Design review of the part shown in the three views and the two pictorial views. Dimensions are in mm from the part's minimum x, y and z. Coordinates: 2 decimals unless noted, no trailing zeros. Write each loop counter-clockwise with the first axis right and the second up, starting at its lowest first coordinate (ties: lowest second). Pieces come first, ordered by that corner, then holes.
Q1. The part is to be moulded in two halves that separate along Y. For the marked faces 1, 2, 3 and 4, say which applies: released by +Y, released by -Y, zero draft, split by the parting line, or undercut.
Q2. For L1, parallel to Y at x = 51, z = 7; L2, parallel to Y at x = 7.95, z = 2.75; L3, parallel to Y at x = 29, z = 51.2, list the stretches that pass through material, from the lowest coordinate up.
Q3. Take a section at B-B, the plane x = 29. Write out the cut boundary in (y, z).
Q4. Take a section at A-A, the plane y = 31. Write out the cut boundary in (x, z), plus the area to 4 significant figures.
Q5. For pin 1 Ø0.9 at (x, y) = (50, 51.5) entering from -Z; pin 2 Ø8 at (x, y) = (44, 18) entering from +Z; pin 3 Ø8 at (x, z) = (34, 32) entering from +Y, all flat-tipped, find the tip position at first contact; note any pin that passes through.
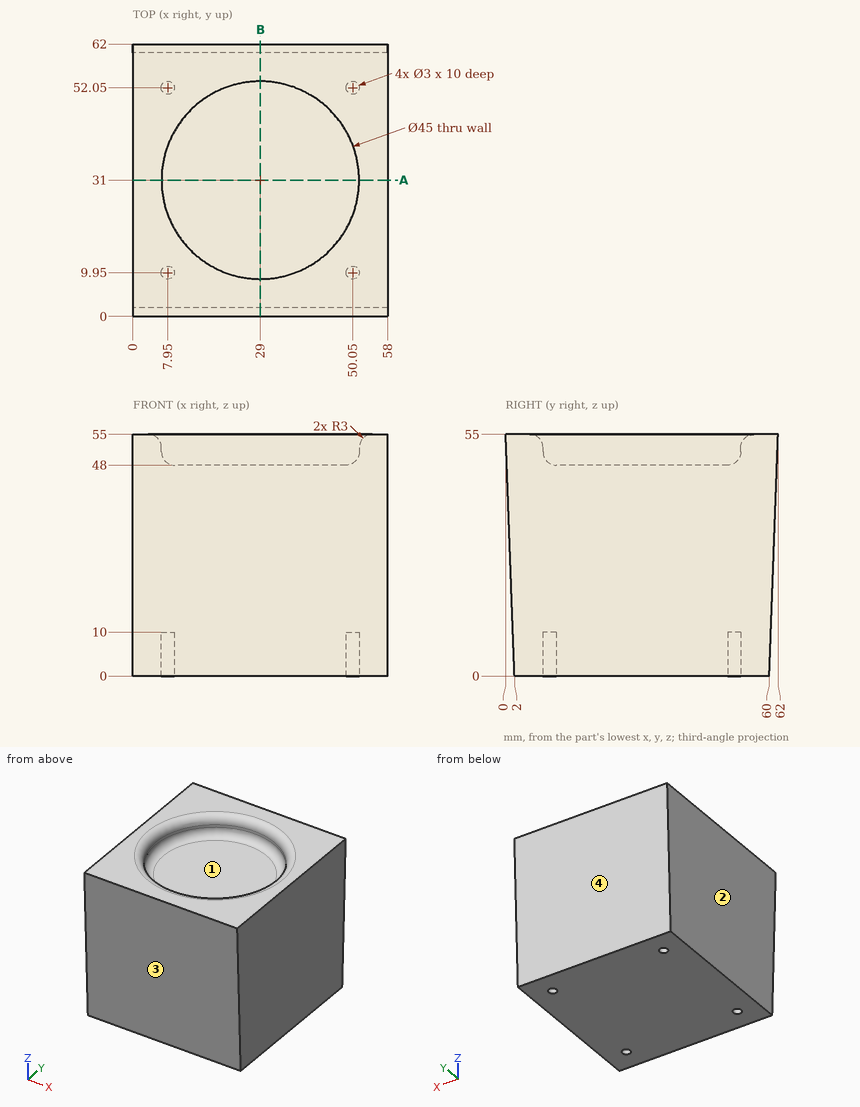
Responses:
1. face 1: undercut
1. face 2: zero draft
1. face 3: released by -Y
1. face 4: released by +Y
2. L1: y = 1.75 to 8.79, 11.11 to 50.89, 53.21 to 60.25
2. L2: y = 1.9 to 8.45, 11.45 to 50.55, 53.55 to 60.1
2. L3: y = 0.14 to 8.5, 53.5 to 61.86
3. outline: (0, 55) - (2, 0) - (60, 0) - (62, 55) - (56.5, 55) arc R3 ccw to (53.5, 52) - (53.5, 51) arc R3 cw to (50.5, 48) - (11.5, 48) arc R3 cw to (8.5, 51) - (8.5, 52) arc R3 ccw to (5.5, 55) - close
4. outline: (0, 0) - (58, 0) - (58, 55) - (54.5, 55) arc R3 ccw to (51.5, 52) - (51.5, 51) arc R3 cw to (48.5, 48) - (9.5, 48) arc R3 cw to (6.5, 51) - (6.5, 52) arc R3 ccw to (3.5, 55) - (0, 55) - close
4. area: 2,875 mm2
5. pin 1: stops at z = 10
5. pin 2: stops at z = 54.51
5. pin 3: stops at y = 61.31
